Build history of the part. All positions in model axes, mm. Coordinates: 2 decimals unless noted, no trailing zeros. Order: outer loops, then holes, each group sorted by start corner. A loop starts at its lowest first (then second) coordinate and runs counter-clockwise, first axis right, second up. Notation, with made-up numbers: (48.25, -20.75) - (91.25, -20.75) arc R22 cw to (91.25, -3.75) - close; hole circle Ø5 at (49.5, -16.75). An arc over 180 degrees is marked (long way). Return JSON: item names as keys, results as strings.
Autodesk Fusion 360 part; units mm, degrees
sketch "Sketch1" plane through (0, 0, 0) normal (0, 0, 1) x (1, 0, 0)
  circle A0 centre (0, 0) radius 31
  dimension "d1" = 62
extrude "Extrude1" add sketch "Sketch1" along normal blind 2
sketch "Sketch2" plane through (0, 0, 2) normal (0, 0, 1) x (-1, 0, 0)
  circle A0 centre (0, 0) radius 31
  circle A1 centre (-7, 0) radius 2.5
  dimension "d5" = 5
extrude "Extrude2" cut sketch "Sketch2" against normal blind 10 contours A1
pattern_circular "C-Pattern1" count 3 over 360 about axis through (0, 0, 1.75) along (0, 0, 1) of "Extrude2"
1. Mould opens along Y. For faces 1 (the cylindrical face through (-2.96, -3.62, 1.01)), 2 (the flat face through (0, 0, 0)), 3 (the cylindrical face through (-4.036, -30.736, 0.986)) say: pulls with the +Y half, pulls with the -Y half, needs draft (parallel to the pull), parting line crosses it, or undercut.
Check values:
{"face 1": "undercut", "face 2": "needs draft", "face 3": "parting line crosses it"}
2. Cut at D-D on y = -13. Give the cut face in (x, z), plus the area to 3 significant figures.
Check values:
{"outline": "(-28.14, 0) - (28.14, 0) - (28.14, 2) - (-28.14, 2) - close", "area": "113 mm²"}
3. Cut at B-B on x = 7. Give the cut face in (y, z), plus the area to 3 significant figures.
Check values:
{"outline": "(-30.2, 0) - (-2.5, 0) - (-2.5, 2) - (-30.2, 2) - close; (2.5, 0) - (30.2, 0) - (30.2, 2) - (2.5, 2) - close", "area": "111 mm²"}
4. Probe L1, parallel to Y at x = -3.5, z = 0.85; L2, parallel to Y at x = 7, z = 0.7; L3, parallel to Y at x = 8.5, z = 1.45. List the from-to ranges inside material, lowest first.
Check values:
{"L1": "-30.8 to -8.56, -3.56 to 3.56, 8.56 to 30.8", "L2": "-30.2 to -2.5, 2.5 to 30.2", "L3": "-29.81 to -2, 2 to 29.81"}
5. Drop a flat-ended pin along its axis: pin 1 (4.5 mm diameter, centred on x = -3.5, y = -6.06, fed in from +Z). Give the stop position or say it passes through.
Check values:
{"pin 1": "through"}
6. Cut at A-A on x = -3.5. Give the cut face in (y, z).
Check values:
{"outline": "(-30.8, 0) - (-8.56, 0) - (-8.56, 2) - (-30.8, 2) - close; (-3.56, 0) - (3.56, 0) - (3.56, 2) - (-3.56, 2) - close; (8.56, 0) - (30.8, 0) - (30.8, 2) - (8.56, 2) - close"}
7. Cut at C-C on z = 1.4. Give the cut face in (x, y), plus the area to 3 significant figures.
Check values:
{"outline": "circle Ø62 at (0, 0); hole circle Ø5 at (-3.5, -6.06); hole circle Ø5 at (-3.5, 6.06); hole circle Ø5 at (7, 0)", "area": "2,960 mm²"}
